Model file for the job. Use its own axes, mm. A direction names the side the tool comes from. Coordinates: 2 decimals unless noted, no trailing zeros. Write each loop counter-clockwise with the first axis right and the second up, starting at its lowest first coordinate (ties: lowest second). Pieces come first, ordered by that corner, then holes. Notation, with made-up numbers: (72, 55) -> (124, 55) arc R21 cw to (124, 73) -> close; hole circle Ø3 at (67, -22.5). An arc over 180 degrees is marked (long way). Answer as a JSON object with one key per item and string values. Group by question number.
from build123d import *

# Parameters (mm, degrees)
F0_W     = 98.044
F0_H     = 98.044
F0_R     = 1.651
F0_R_2   = 2.286
F0_R_3   = 2.032
F0_R_4   = 1.397
F1_DEPTH = 1.5875
F2_DEPTH = 5.08


with BuildPart() as f1:
    # F0 (on Top) → F1 (new body)
    with BuildSketch(Plane.XY):
        Rectangle(F0_W, F0_H)
        with Locations((-45.847, -45.847)):
            Circle(F0_R, mode=Mode.SUBTRACT)
        with Locations((-37.338, -7.874)):
            Circle(F0_R_2, mode=Mode.SUBTRACT)
        with Locations((-0.254, -16.51)):
            Circle(F0_R_3, mode=Mode.SUBTRACT)
        with Locations((45.847, -45.847)):
            Circle(F0_R, mode=Mode.SUBTRACT)
        with Locations((9.017, -16.51)):
            Circle(F0_R_3, mode=Mode.SUBTRACT)
        with Locations((19.05, -16.51)):
            Circle(F0_R_3, mode=Mode.SUBTRACT)
        with Locations((28.448, -20.32)):
            Circle(F0_R_3, mode=Mode.SUBTRACT)
        with Locations((28.448, -13.716)):
            Circle(F0_R_3, mode=Mode.SUBTRACT)
        with Locations((37.8543436527, -16.51)):
            Circle(F0_R_3, mode=Mode.SUBTRACT)
        with Locations((37.338, -7.874)):
            Circle(F0_R_2, mode=Mode.SUBTRACT)
        with Locations((-45.847, 45.847)):
            Circle(F0_R, mode=Mode.SUBTRACT)
        with BuildLine():
            Line((-7.9581705729, 39.497), (-8.5479709201, 39.497))
            Line((-8.5479709201, 39.497), (-10.6839301215, 45.0780546875))
            Line((-10.6839301215, 45.0780546875), (-10.7183810764, 45.0780546875))
            add(Edge.make_bspline(
                [(-10.7183810764, 45.0780546875), (-10.6577473958, 44.415218316), (-10.6577473958, 43.5015789931)],
                knots=[0, 0, 0, 1, 1, 1], degree=2))
            Line((-10.6577473958, 43.5015789931), (-10.6577473958, 39.497))
            Line((-10.6577473958, 39.497), (-11.3343641493, 39.497))
            Line((-11.3343641493, 39.497), (-11.3343641493, 45.7932565104))
            Line((-11.3343641493, 45.7932565104), (-10.2319335938, 45.7932565104))
            Line((-10.2319335938, 45.7932565104), (-8.2379123264, 40.5994305556))
            Line((-8.2379123264, 40.5994305556), (-8.2034613715, 40.5994305556))
            Line((-8.2034613715, 40.5994305556), (-6.1929036458, 45.7932565104))
            Line((-6.1929036458, 45.7932565104), (-5.0987413194, 45.7932565104))
            Line((-5.0987413194, 45.7932565104), (-5.0987413194, 39.497))
            Line((-5.0987413194, 39.497), (-5.8304796007, 39.497))
            Line((-5.8304796007, 39.497), (-5.8304796007, 43.5539444444))
            add(Edge.make_bspline(
                [(-5.8304796007, 43.5539444444), (-5.8304796007, 44.2512317708), (-5.7698459201, 45.0697864583)],
                knots=[0, 0, 0, 1, 1, 1], degree=2))
            Line((-5.7698459201, 45.0697864583), (-5.804296875, 45.0697864583))
            Line((-5.804296875, 45.0697864583), (-7.9581705729, 39.497))
        make_face(mode=Mode.SUBTRACT)
        with BuildLine():
            Line((1.5461588542, 45.7932565104), (1.5461588542, 39.497))
            Line((1.5461588542, 39.497), (0.7110677083, 39.497))
            Line((0.7110677083, 39.497), (-2.7298936632, 44.7803984375))
            Line((-2.7298936632, 44.7803984375), (-2.7643446181, 44.7803984375))
            add(Edge.make_bspline(
                [(-2.7643446181, 44.7803984375), (-2.6954427083, 43.8502226563), (-2.6954427083, 43.075765191)],
                knots=[0, 0, 0, 1, 1, 1], degree=2))
            Line((-2.6954427083, 43.075765191), (-2.6954427083, 39.497))
            Line((-2.6954427083, 39.497), (-3.3720594618, 39.497))
            Line((-3.3720594618, 39.497), (-3.3720594618, 45.7932565104))
            Line((-3.3720594618, 45.7932565104), (-2.5452365451, 45.7932565104))
            Line((-2.5452365451, 45.7932565104), (0.8874565972, 40.5305286458))
            Line((0.8874565972, 40.5305286458), (0.9219075521, 40.5305286458))
            add(Edge.make_bspline(
                [(0.9219075521, 40.5305286458), (0.9136393229, 40.6462838542), (0.8833224826, 41.2774253472)],
                knots=[0, 0, 0, 1, 1, 1], degree=2))
            add(Edge.make_bspline(
                [(0.8833224826, 41.2774253472), (0.8530056424, 41.9085668403), (0.8612738715, 42.1800403646)],
                knots=[0, 0, 0, 1, 1, 1], degree=2))
            Line((0.8612738715, 42.1800403646), (0.8612738715, 45.7932565104))
            Line((0.8612738715, 45.7932565104), (1.5461588542, 45.7932565104))
        make_face(mode=Mode.SUBTRACT)
        with BuildLine():
            ThreePointArc((-35.814, 21.1561162011), (-39.4248229441, 23.793255592), (-35.052, 22.86))
            ThreePointArc((-35.052, 22.86), (-35.2024819874, 22.0443047028), (-35.6341162011, 21.336))
            Line((-35.6341162011, 21.336), (35.6341162011, 21.336))
            ThreePointArc((35.6341162011, 21.336), (36.5223047028, 24.9955180126), (39.624, 22.86))
            ThreePointArc((39.624, 22.86), (38.271255592, 20.7731770559), (35.814, 21.1561162011))
            Line((35.814, 21.1561162011), (35.814, -5.588))
            Line((35.814, -5.588), (-35.814, -5.588))
            Line((-35.814, -5.588), (-35.814, 21.1561162011))
        make_face(mode=Mode.SUBTRACT)
        with BuildLine():
            add(Edge.make_bspline(
                [(6.4574869792, 42.2227595486), (6.8295572917, 41.8176163194), (6.8295572917, 41.1726944444)],
                knots=[0, 0, 0, 1, 1, 1], degree=2))
            add(Edge.make_bspline(
                [(6.8295572917, 41.1726944444), (6.8295572917, 40.3417374132), (6.2266655816, 39.8759605035)],
                knots=[0, 0, 0, 1, 1, 1], degree=2))
            add(Edge.make_bspline(
                [(6.2266655816, 39.8759605035), (5.6237738715, 39.4101835938), (4.5902452257, 39.4101835938)],
                knots=[0, 0, 0, 1, 1, 1], degree=2))
            add(Edge.make_bspline(
                [(4.5902452257, 39.4101835938), (3.4712782118, 39.4101835938), (2.8676974826, 39.6995716146)],
                knots=[0, 0, 0, 1, 1, 1], degree=2))
            Line((2.8676974826, 39.6995716146), (2.8676974826, 40.4051271701))
            add(Edge.make_bspline(
                [(2.8676974826, 40.4051271701), (3.2563042535, 40.2425186632), (3.7124348958, 40.1474340278)],
                knots=[0, 0, 0, 1, 1, 1], degree=2))
            add(Edge.make_bspline(
                [(3.7124348958, 40.1474340278), (4.1685655382, 40.0523493924), (4.6164279514, 40.0523493924)],
                knots=[0, 0, 0, 1, 1, 1], degree=2))
            add(Edge.make_bspline(
                [(4.6164279514, 40.0523493924), (5.3481662326, 40.0523493924), (5.7188585069, 40.3300240885)],
                knots=[0, 0, 0, 1, 1, 1], degree=2))
            add(Edge.make_bspline(
                [(5.7188585069, 40.3300240885), (6.0895507813, 40.6076987847), (6.0895507813, 41.1037925347)],
                knots=[0, 0, 0, 1, 1, 1], degree=2))
            add(Edge.make_bspline(
                [(6.0895507813, 41.1037925347), (6.0895507813, 41.4303875868), (5.9579481337, 41.6391603733)],
                knots=[0, 0, 0, 1, 1, 1], degree=2))
            add(Edge.make_bspline(
                [(5.9579481337, 41.6391603733), (5.8263454861, 41.8479331597), (5.5183539497, 42.0250110677)],
                knots=[0, 0, 0, 1, 1, 1], degree=2))
            add(Edge.make_bspline(
                [(5.5183539497, 42.0250110677), (5.2103624132, 42.2020889757), (4.5819769965, 42.4253311632)],
                knots=[0, 0, 0, 1, 1, 1], degree=2))
            add(Edge.make_bspline(
                [(4.5819769965, 42.4253311632), (3.7041666667, 42.7395238715), (3.3272732205, 43.1701608073)],
                knots=[0, 0, 0, 1, 1, 1], degree=2))
            add(Edge.make_bspline(
                [(3.3272732205, 43.1701608073), (2.9503797743, 43.6007977431), (2.9503797743, 44.2939509549)],
                knots=[0, 0, 0, 1, 1, 1], degree=2))
            add(Edge.make_bspline(
                [(2.9503797743, 44.2939509549), (2.9503797743, 45.0215551215), (3.4967719184, 45.4521920573)],
                knots=[0, 0, 0, 1, 1, 1], degree=2))
            add(Edge.make_bspline(
                [(3.4967719184, 45.4521920573), (4.0431640625, 45.8828289931), (4.9444010417, 45.8828289931)],
                knots=[0, 0, 0, 1, 1, 1], degree=2))
            add(Edge.make_bspline(
                [(4.9444010417, 45.8828289931), (5.8828450521, 45.8828289931), (6.6710828993, 45.5383194444)],
                knots=[0, 0, 0, 1, 1, 1], degree=2))
            Line((6.6710828993, 45.5383194444), (6.442328559, 44.9016657986))
            add(Edge.make_bspline(
                [(6.442328559, 44.9016657986), (5.662358941, 45.2282608507), (4.9264865451, 45.2282608507)],
                knots=[0, 0, 0, 1, 1, 1], degree=2))
            add(Edge.make_bspline(
                [(4.9264865451, 45.2282608507), (4.3449544271, 45.2282608507), (4.0176703559, 44.9788359375)],
                knots=[0, 0, 0, 1, 1, 1], degree=2))
            add(Edge.make_bspline(
                [(4.0176703559, 44.9788359375), (3.6903862847, 44.7294110243), (3.6903862847, 44.2856827257)],
                knots=[0, 0, 0, 1, 1, 1], degree=2))
            add(Edge.make_bspline(
                [(3.6903862847, 44.2856827257), (3.6903862847, 43.9590876736), (3.8109646267, 43.7496258681)],
                knots=[0, 0, 0, 1, 1, 1], degree=2))
            add(Edge.make_bspline(
                [(3.8109646267, 43.7496258681), (3.9315429688, 43.5401640625), (4.2181749132, 43.3658422309)],
                knots=[0, 0, 0, 1, 1, 1], degree=2))
            add(Edge.make_bspline(
                [(4.2181749132, 43.3658422309), (4.5048068576, 43.1915203993), (5.0946072049, 42.9806805556)],
                knots=[0, 0, 0, 1, 1, 1], degree=2))
            add(Edge.make_bspline(
                [(5.0946072049, 42.9806805556), (6.0854166667, 42.6279027778), (6.4574869792, 42.2227595486)],
                knots=[0, 0, 0, 1, 1, 1], degree=2))
        make_face(mode=Mode.SUBTRACT)
        Polygon((11.6278862847, 39.497), (8.1180230035, 39.497), (8.1180230035, 45.7932565104), (8.8497612847, 45.7932565104), (8.8497612847, 40.1598363715), (11.6278862847, 40.1598363715), align=None, mode=Mode.SUBTRACT)
        with Locations((45.847, 45.847)):
            Circle(F0_R, mode=Mode.SUBTRACT)
        with Locations((-37.338, -7.874)):
            Circle(F0_R_2)
        with Locations((-37.338, -7.874)):
            Circle(F0_R_4, mode=Mode.SUBTRACT)
        with Locations((37.338, -7.874)):
            Circle(F0_R_2)
        with Locations((37.338, -7.874)):
            Circle(F0_R_4, mode=Mode.SUBTRACT)
        with BuildLine():
            ThreePointArc((39.624, 22.86), (36.5223047028, 24.9955180126), (35.6341162011, 21.336))
            Line((35.6341162011, 21.336), (35.814, 21.336))
            Line((35.814, 21.336), (35.814, 21.1561162011))
            ThreePointArc((35.814, 21.1561162011), (38.271255592, 20.7731770559), (39.624, 22.86))
        make_face()
        with Locations((37.338, 22.86)):
            Circle(F0_R_4, mode=Mode.SUBTRACT)
        with BuildLine():
            ThreePointArc((-35.6341162011, 21.336), (-35.2024819874, 22.0443047028), (-35.052, 22.86))
            ThreePointArc((-35.052, 22.86), (-39.4248229441, 23.793255592), (-35.814, 21.1561162011))
            Line((-35.814, 21.1561162011), (-35.814, 21.336))
            Line((-35.814, 21.336), (-35.6341162011, 21.336))
        make_face()
        with Locations((-37.338, 22.86)):
            Circle(F0_R_4, mode=Mode.SUBTRACT)
    extrude(amount=F1_DEPTH)

    # F0 (on Top) → F2 (join)
    with BuildSketch(Plane.XY):
        with BuildLine():
            ThreePointArc((39.624, 22.86), (36.5223047028, 24.9955180126), (35.6341162011, 21.336))
            Line((35.6341162011, 21.336), (35.814, 21.336))
            Line((35.814, 21.336), (35.814, 21.1561162011))
            ThreePointArc((35.814, 21.1561162011), (38.271255592, 20.7731770559), (39.624, 22.86))
        make_face()
        with Locations((37.338, 22.86)):
            Circle(F0_R_4, mode=Mode.SUBTRACT)
        with Locations((-37.338, -7.874)):
            Circle(F0_R_2)
        with Locations((-37.338, -7.874)):
            Circle(F0_R_4, mode=Mode.SUBTRACT)
        with BuildLine():
            ThreePointArc((-35.6341162011, 21.336), (-35.2024819874, 22.0443047028), (-35.052, 22.86))
            ThreePointArc((-35.052, 22.86), (-39.4248229441, 23.793255592), (-35.814, 21.1561162011))
            Line((-35.814, 21.1561162011), (-35.814, 21.336))
            Line((-35.814, 21.336), (-35.6341162011, 21.336))
        make_face()
        with Locations((-37.338, 22.86)):
            Circle(F0_R_4, mode=Mode.SUBTRACT)
        with Locations((37.338, -7.874)):
            Circle(F0_R_2)
        with Locations((37.338, -7.874)):
            Circle(F0_R_4, mode=Mode.SUBTRACT)
    extrude(amount=-F2_DEPTH)


solid = f1.part
(1) Cut at D-D on x = -15.5. List the corners of the cut face in (y, z), plus the area to 3 significant figures.
(2) Cut at C-C on z = -3. List the corners of the cut face in (x, y) (3 decimals), plus the area to 3 significant figures.
(3) Cut at B-B on x = 19.05. List the corners of the cut face in (y, z).
(4) 3-axis set-ups, long thin cutter, end or side, ignore diameter. For faces 1 (the face through (0, 21.336, 1)), 2 (the face through (-36, 24, -5.08)), 3 (the face through (-35.158, -7.187, -2.504)): which of +Z, -Z, +X, -X, +Y, -Y reach the whole face in a straight line?
(5) Cut at A-A on y = -1. List the corners of the cut face in (x, z).
(6) Wall check: probe 1 along Y at (x, z) = (2, 1.25); probe 2 along Y at (x, z) = (30, 1); probe 3 along Z at (x, y) = (-31.5, -36). Give the ranges that are in metal, low to high.
(7) Pull direction X, two halves, no side cores. Call faces 4 (the face through (35.814, 8, 1)), 5 (the face through (-36, -7, -5.08)): released by +X, released by -X, zero draft, split by the parting line, or undercut.
(8) Pin check, flat tips, straight feed: pin 1 (12 mm diameter, centred on x = -27.5, y = 10, fed in from -Z); pin 2 (4 mm diameter, centred on y = -6.5, z = -0.5, fed in from -X); pin 3 (1 mm diameter, centred on x = 34.5, y = 34, fed in from -Z). Stop position of each tip, or through.
Results found:
{
 "1": {"outline": "(-49.02, 0) -> (-5.59, 0) -> (-5.59, 1.59) -> (-49.02, 1.59) -> close; (21.34, 0) -> (49.02, 0) -> (49.02, 1.59) -> (21.34, 1.59) -> close", "area": "113 mm²"},
 "2": {"outline": "circle Ø4.572 at (-37.338, -7.874); (-35.814, 21.156) -> (-35.814, 21.336) -> (-35.634, 21.336) arc R2.286 ccw (long way) to start; circle Ø4.572 at (37.338, -7.874); (35.634, 21.336) -> (35.814, 21.336) -> (35.814, 21.156) arc R2.286 ccw (long way) to start; hole circle Ø2.794 at (-37.338, -7.874); hole circle Ø2.794 at (-37.338, 22.86); hole circle Ø2.794 at (37.338, -7.874); hole circle Ø2.794 at (37.338, 22.86)", "area": "41.1 mm²"},
 "3": {"outline": "(-49.02, 0) -> (-18.54, 0) -> (-18.54, 1.59) -> (-49.02, 1.59) -> close; (-14.48, 0) -> (-5.59, 0) -> (-5.59, 1.59) -> (-14.48, 1.59) -> close; (21.34, 0) -> (49.02, 0) -> (49.02, 1.59) -> (21.34, 1.59) -> close"},
 "4": {"face 1": "+Z, -Z", "face 2": "-Z, +X, -X, +Y, -Y", "face 3": "-Z"},
 "5": {"outline": "(-49.02, 0) -> (-35.81, 0) -> (-35.81, 1.59) -> (-49.02, 1.59) -> close; (35.81, 0) -> (49.02, 0) -> (49.02, 1.59) -> (35.81, 1.59) -> close"},
 "6": {"probe 1": "y = -49.02 to -5.59, 21.34 to 49.02", "probe 2": "y = -49.02 to -21.63, -19.01 to -15.03, -12.4 to -5.59, 21.34 to 49.02", "probe 3": "z = 0 to 1.59"},
 "7": {"face 4": "undercut", "face 5": "zero draft"},
 "8": {"pin 1": "passes through", "pin 2": "stops at x = -49.02", "pin 3": "stops at z = 0"}
}
